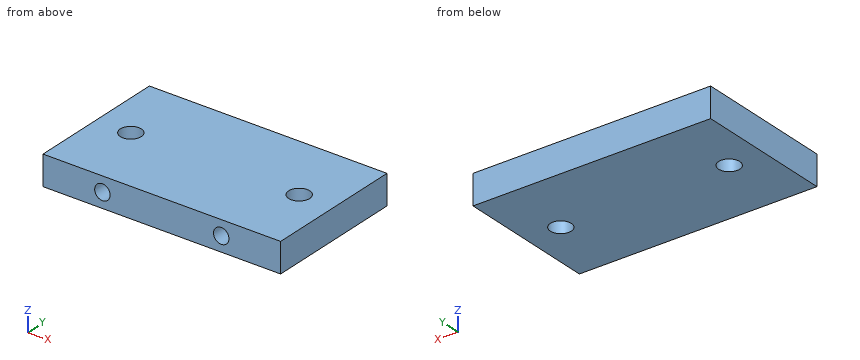
from build123d import *

# Parameters (mm, degrees)
SKETCH1_W                 = 50.8
SKETCH1_H                 = 30
SKETCH1_R                 = 2.25
BOSS_EXTRUDE1_DEPTH       = 6.35
M4X0_7_TAPPED_HOLE1_D     = 3.3
M4X0_7_TAPPED_HOLE1_DEPTH = 14.732
M4X0_7_TAPPED_HOLE1_TIP   = 0.991420021


with BuildPart() as part:
    # Sketch1 → Boss-Extrude1 (new body)
    with BuildSketch(Plane.XY):
        with Locations((25.4, 15)):
            Rectangle(SKETCH1_W, SKETCH1_H)
        with Locations((7.400000059, 15)):
            Circle(SKETCH1_R, mode=Mode.SUBTRACT)
        with Locations((43.400000059, 15)):
            Circle(SKETCH1_R, mode=Mode.SUBTRACT)
    extrude(amount=BOSS_EXTRUDE1_DEPTH)

    # M4x0.7 Tapped Hole1
    with Locations(Plane(origin=(0, 0, 0), x_dir=(-1, 0, 0), z_dir=(0, -1, 0))):
        with Locations((-12.7, -3.175), (-38.1, -3.175)):
            Hole(M4X0_7_TAPPED_HOLE1_D / 2, depth=M4X0_7_TAPPED_HOLE1_DEPTH)
            with Locations((0, 0, -(M4X0_7_TAPPED_HOLE1_DEPTH + M4X0_7_TAPPED_HOLE1_TIP / 2))):  # 118° drill point
                Cone(0, M4X0_7_TAPPED_HOLE1_D / 2, M4X0_7_TAPPED_HOLE1_TIP, mode=Mode.SUBTRACT)


solid = part.part
Source: CAD feature listing. Evaluate the final solid. Frame: model axes, mm. Coordinates: 2 decimals unless noted, no trailing zeros. Loops run counter-clockwise (first coordinate to the right, second up) from the corner with the lowest first, then second, coordinate; pieces in that order, holes last. Notation, with made-up numbers: (-3, 61) - (45, 61) arc R22 ccw to (45, 81) - close; hole circle Ø7 at (78, -14). An arc over 180 degrees is marked (long way). Return JSON: item names as keys, results as strings.
Q1. Contact query for flat-ended pins moving along their axis: P1, Ø2.5, axis at x = 38.1, z = 3.175, coming from the -Y side; P2, Ø3.5, axis at x = 7.4, y = 15, coming from the -Z side. Output: stop coordinate, or through.
Results:
{"P1": "y = 14.97", "P2": "through"}
Q2. Material intervals for line 1 along Y through (x, z) = (7.4, 3.5); line 2 along X through (y, z) = (6, 4.25); line 3 along Z through (x, y) = (38.1, 8) (3 decimals), sorted ascending.
Results:
{"line 1": "0 to 12.75, 17.25 to 30", "line 2": "0 to 11.45, 13.95 to 36.85, 39.35 to 50.8", "line 3": "0 to 1.525, 4.825 to 6.35"}
Q3. Section B-B, the plane y = 7.25. Return loops of the section in (x, z) (3 decimals).
Results:
{"outline": "(0, 0) - (50.8, 0) - (50.8, 6.35) - (0, 6.35) - close; hole circle Ø3.3 at (12.7, 3.175); hole circle Ø3.3 at (38.1, 3.175)"}
Q4. Section A-A, the plane x = 43.4. Return loops of the section in (y, z), plus the area to 3 significant figures.
Results:
{"outline": "(0, 0) - (12.75, 0) - (12.75, 6.35) - (0, 6.35) - close; (17.25, 0) - (30, 0) - (30, 6.35) - (17.25, 6.35) - close", "area": "162 mm2"}
Q5. Section C-C, the plane z = 2. Give the number of separate pieces and of enclosed holes in the cut face, plus the area to 3 significant figures.
Results:
{"separate pieces": "1", "enclosed holes": "2", "area": "1,420 mm2"}
